from build123d import *

# Parameters (mm, degrees)
SKETCH_1_W          = 30
SKETCH_1_H          = 133
EXTRUDE_1_DEPTH     = 6
CHAMFER_1_SIZE      = 10
SKETCH_2_R          = 6
CUT_EXTRUDE_1_DEPTH = 134.97761007


with BuildPart() as part:
    # Эскиз1 → Бобышка-Вытянуть1 (new body)
    with BuildSketch(Plane.XY):
        with Locations((0, -66.5)):
            Rectangle(SKETCH_1_W, SKETCH_1_H)
    extrude(amount=-EXTRUDE_1_DEPTH)

    # Фаска1
    chamfer_1_edges = [part.edges().sort_by_distance(p)[0] for p in [
        (15, -133, -3),
        (-15, -133, -3),
    ]]
    chamfer(chamfer_1_edges, length=CHAMFER_1_SIZE)

    # Эскиз2 → Вырез-Вытянуть1 (cut, through all)
    with BuildSketch(Plane.XY):
        with Locations((0, -121)):
            Circle(SKETCH_2_R)
    extrude(amount=-CUT_EXTRUDE_1_DEPTH, mode=Mode.SUBTRACT)


solid = part.part
Can you work these out from the model? Positions are in its coordinate system, mm. Give positions to 0.01 mm unless a question says otherwise; leave off trailing zeros. Loops run counter-clockwise (first coordinate to the right, second up) from the corner with the lowest first, then second, coordinate; pieces in that order, holes last. Notation, with made-up numbers: (61, -1.75) - (88, -1.75) arc R14 cw to (88, 4.25) - close; hole circle Ø7 at (47, 13.5). An arc over 180 degrees is marked (long way). One line per item, written item: value.
(1) I'm going to push flat-ended pins straight in: pin 1 (1 mm diameter, centred on x = 11, z = -3.5, fed in from -Y); pin 2 (11 mm diameter, centred on x = 0, y = -121, fed in from -Z). Where does each tip first touch, or does it pass through?
Verdict:
pin 1: y = -127.5
pin 2: through
(2) If we section it at D-D, the plane x = -11.75: List the corners of the cut face in (y, z) for me.
Verdict:
outline: (-126.25, -6) - (0, -6) - (0, 0) - (-126.25, 0) - close
(3) I need wall thicknesses on line 1 along Y through (x, z) = (0, -1.15); line 2 along Y through (x, z) = (11, -1.05); line 3 along X through (y, z) = (-124.5, -1.7). Which ranges of each line are inside material? Lowest first, please.
Verdict:
line 1: -133 to -127, -115 to 0
line 2: -127 to 0
line 3: -13.5 to -4.87, 4.87 to 13.5
(4) If we section it at B-B, the plane y = -121: List the corners of the cut face in (x, z) for me, plus the area to 3 significant figures.
Verdict:
outline: (-15, -6) - (-6, -6) - (-6, 0) - (-15, 0) - close; (6, -6) - (15, -6) - (15, 0) - (6, 0) - close
area: 108 mm^2
(5) If we section it at A-A, the plane x = 0: List the corners of the cut face in (y, z) for me.
Verdict:
outline: (-133, -6) - (-127, -6) - (-127, 0) - (-133, 0) - close; (-115, -6) - (0, -6) - (0, 0) - (-115, 0) - close
(6) If we mould it in two halves opening along Y, with no side actions, what happens to faces 1 (the face through (0, -133, -3)), 2 (the face through (15, -62, -3)), 3 (the face through (-0.78, -115.05, -2.96)), 4 (the face through (0, 0, -3))? For each: released by +Y, released by -Y, zero draft, split by the parting line, or undercut.
Verdict:
face 1: released by -Y
face 2: zero draft
face 3: undercut
face 4: released by +Y
(7) If we section it at C-C, the plane z = -2.55: List the corners of the cut face in (x, y) for me, plus the area to 3 significant figures.
Verdict:
outline: (-15, -123) - (-5, -133) - (5, -133) - (15, -123) - (15, 0) - (-15, 0) - close; hole circle Ø12 at (0, -121)
area: 3,780 mm^2
